Here's the drawing with two shaded views (mm, measured from the low corner). I have some questions. A direction names the side the tool comes from. Round coordinates to 2 decimals unless told otherwise and drop trailing zeros. Order: outer loops, then holes, each group sorted by start corner. A loop starts at its lowest first (then second) coordinate and runs counter-clockwise, first axis right, second up. Notation, with made-up numbers: (-5, 83.5) - (29, 83.5) arc R16 ccw to (29, 113.5) - close; hole circle Ø8 at (26.25, 69.5). An arc over 180 degrees is marked (long way). One line per item, written item: value.
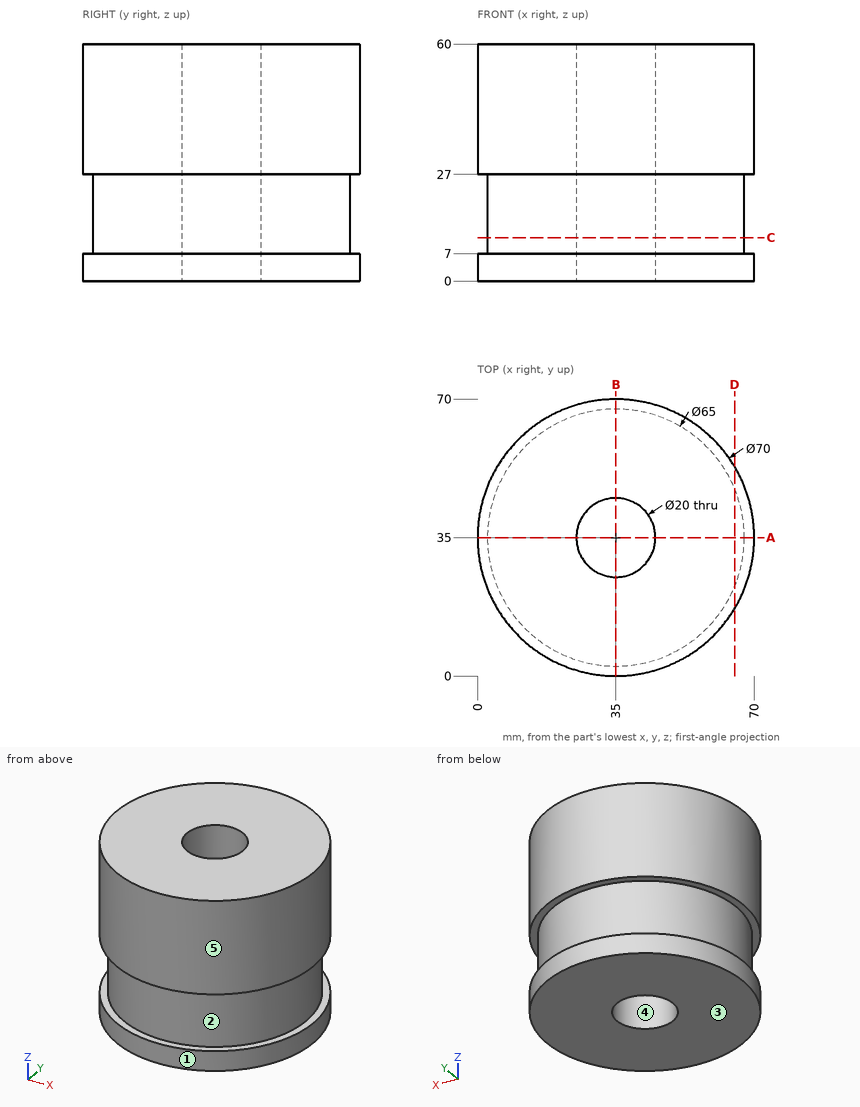
Q1. If we section it at D-D, the plane x = 65: Please give me the cut outline in (y, z), then the cut area to 3 significant figures.
Results list:
outline: (16.97, 0) - (53.03, 0) - (53.03, 7) - (47.5, 7) - (47.5, 27) - (53.03, 27) - (53.03, 60) - (16.97, 60) - (16.97, 27) - (22.5, 27) - (22.5, 7) - (16.97, 7) - close
area: 1,940 mm²
Q2. If we section it at C-C, the plane z = 11: Please give me the cut outline in (x, y), then the cut area to 3 significant figures.
Results list:
outline: circle Ø65 at (35, 35); hole circle Ø20 at (35, 35)
area: 3,000 mm²
Q3. If we section it at A-A, the plane y = 35: Please give me the cut outline in (x, z).
Results list:
outline: (0, 0) - (25, 0) - (25, 60) - (0, 60) - (0, 27) - (2.5, 27) - (2.5, 7) - (0, 7) - close; (45, 0) - (70, 0) - (70, 7) - (67.5, 7) - (67.5, 27) - (70, 27) - (70, 60) - (45, 60) - close
Q4. We'd pull the mould along X, two halves only. Please class the marked faces 3, 4 and 5: released by +X, released by -X, zero draft, split by the parting line, or undercut.
Results list:
face 3: zero draft
face 4: undercut
face 5: split by the parting line
Q5. If I drill on line 1 along Y through (x, z) = (35, 18.5); line 2 along Z through (x, y) = (56, 62); line 3 along Y through (x, z) = (35, 44), over which ranges is the centre line in solid material (lowest first)?
Results list:
line 1: 2.5 to 25, 45 to 67.5
line 2: 0 to 7, 27 to 60
line 3: 0 to 25, 45 to 70
Q6. Which directions (+Z, -Z, +X, -X, +Y, -Y) give clear straight access to the entire face, cutting with the end or side of a thin tool? Please do the marked faces 1 and 2.
Results list:
face 1: +Z, -Z
face 2: none
Q7. Will these pins go through, and if not, where does the flat tip stop? pin 1 (8 mm diameter, centred on y = 16.5, z = 27, fed in from -X); pin 2 (8 mm diameter, centred on x = 17, z = 20, fed in from -Y); pin 3 (2 mm diameter, centred on x = 56, z = 51, fed in from +Y).
Results list:
pin 1: x = 3.14
pin 2: y = 5.67
pin 3: y = 63.72
